from build123d import *

# Parameters (mm, degrees)
BOSS_EXTRUDE1_DEPTH = 19.05
BOSS_EXTRUDE2_DEPTH = 19.05


with BuildPart() as part:
    # Sketch1 → Boss-Extrude1 (new body)
    with BuildSketch(Plane.XY):
        with BuildLine():
            Line((-2.38125, 7.571892411), (-2.38125, 5.55625))
            Line((-2.38125, 5.55625), (2.38125, 5.55625))
            Line((2.38125, 5.55625), (2.38125, 7.571892411))
            ThreePointArc((2.38125, 7.571892411), (0, -7.9375), (-2.38125, 7.571892411))
        make_face()
    extrude(amount=BOSS_EXTRUDE1_DEPTH)

    # Sketch2 → Boss-Extrude2 (add)
    with BuildSketch(Plane.XY.offset(19.05)):
        with BuildLine():
            Line((-1.5875, 6.148361062), (-1.5875, 4.7625))
            Line((-1.5875, 4.7625), (1.5875, 4.7625))
            Line((1.5875, 4.7625), (1.5875, 6.148361062))
            ThreePointArc((1.5875, 6.148361062), (0, -6.35), (-1.5875, 6.148361062))
        make_face()
    extrude(amount=BOSS_EXTRUDE2_DEPTH)


solid = part.part
Geometry check sheet. Reference: the model listing, model coordinates, mm. A direction names the side the tool comes from. Give positions to 0.01 mm unless a question says otherwise; leave off trailing zeros. Loops run counter-clockwise (first coordinate to the right, second up) from the corner with the lowest first, then second, coordinate; pieces in that order, holes last. Notation, with made-up numbers: M 7.25,40 L 43.25,40 A28 cw 43.25,59 Z; hole C 26.25,-0.5 d8. An arc over 180 degrees is marked long. Answer as a JSON object with one key per item and string values. Group by question number.
Item 1: Material ranges on L1, parallel to Z at x = -3, y = -6.25; L2, parallel to X at y = 0.25, z = 4.5; L3, parallel to X at y = 5.5, z = 23.5, recorded low to high.
Item 2: Access from +Z, -Z, +X, -X, +Y, -Y to the whole of each face (thin tool, end or side, straight path). Record for faces 5 (the flat face through (0, 0, 38.1)), 6 (the cylindrical face through (0.257, -6.345, 28.442)), 7 (the flat face through (0, 4.762, 28)).
Item 3: Sectioned sample at B-B on x = 0. Record the boundary of the cut face in (y, z).
Item 4: Sectioned sample at A-A on y = 0. Record the boundary of the cut face in (x, z).
Item 5: Mould release check, pull along X, two halves, no side actions. Record for faces 1 (the flat face through (-0.6, -6.5, 19.05)), 2 (the flat face through (0, 5.556, 9)), 3 (the flat face through (2.381, 7, 9)), 4 (the cylindrical face through (0.32, -7.93, 9.39)): pulls with the +X half, pulls with the -X half, needs draft (parallel to the pull), parting line crosses it, or undercut.
Item 6: Sectioned sample at C-C on z = 25. Record the boundary of the cut face in (x, y).
Item 7: Gauge pin test, flat ends, axial feed: pin 1 (6 mm diameter, centred on y = -3, z = 32.5, fed in from -X); pin 2 (0.7 mm diameter, centred on x = -2, y = 6, fed in from -Z); pin 3 (1 mm diameter, centred on y = 6, z = 10.5, fed in from -X). Record the tip position at first contact, or that the pin passes through.
Item 8: Sectioned sample at D-D on z = 15.5. Record the boundary of the cut face in (x, y) (1 decimal), plus the area to 3 significant figures.
Findings below:
{
 "1": {"L1": "0 to 19.05", "L2": "-7.93 to 7.93", "L3": "-3.17 to -1.59, 1.59 to 3.17"},
 "2": {"face 5": "+Z, +X, -X, +Y, -Y", "face 6": "+Z", "face 7": "+Z, +Y"},
 "3": {"outline": "M -7.94,0 L 5.56,0 L 5.56,19.05 L 4.76,19.05 L 4.76,38.1 L -6.35,38.1 L -6.35,19.05 L -7.94,19.05 Z"},
 "4": {"outline": "M -7.94,0 L 7.94,0 L 7.94,19.05 L 6.35,19.05 L 6.35,38.1 L -6.35,38.1 L -6.35,19.05 L -7.94,19.05 Z"},
 "5": {"face 1": "needs draft", "face 2": "undercut", "face 3": "undercut", "face 4": "parting line crosses it"},
 "6": {"outline": "M -1.59,4.76 L -1.59,6.15 A6.35 ccw long 1.59,6.15 L 1.59,4.76 Z"},
 "7": {"pin 1": "x = -6.35", "pin 2": "z = 19.05", "pin 3": "x = -5.72"},
 "8": {"outline": "M -2.4,5.6 L -2.4,7.6 A7.9 ccw long 2.4,7.6 L 2.4,5.6 Z", "area": "187 mm2"}
}
